from build123d import *

# Parameters (mm, degrees)
SKETCH024_W             = 144.5
SKETCH024_H             = 350
PAD017_DEPTH            = 19
FILLET007_R             = 20
SKETCH025_R             = 2
POCKET015_DEPTH         = 19.001
CHAMFER005_SIZE         = 5
POCKET020_DEPTH         = 19.001
CHAMFER006_SIZE         = 5
CHAMFER007_SIZE         = 3
SKETCH045_W             = 131
SKETCH045_H             = 20
POCKET029_DEPTH         = 14
BODY013_PLACEMENT_ANGLE = 180


with BuildPart() as part:
    # Sketch024 → Pad017 (new body)
    with BuildSketch(Plane.XY):
        with Locations((307.25, 41.2)):
            Rectangle(SKETCH024_W, SKETCH024_H)
    extrude(amount=PAD017_DEPTH)

    # Fillet007
    fillet007_edges = [part.edges().sort_by_distance(p)[0] for p in [
        (379.5, 216.2, 9.5),
        (379.5, -133.8, 9.5),
    ]]
    fillet(fillet007_edges, radius=FILLET007_R)

    # Sketch025 (on Face5 of Fillet007) → Pocket015 (cut, through all)
    with BuildSketch(Plane.XY.offset(19)):
        with Locations((359.5, 196.2)):
            Circle(SKETCH025_R)
        with Locations((359.5, -113.8)):
            Circle(SKETCH025_R)
        with Locations((255, -113.8)):
            Circle(SKETCH025_R)
        with Locations((255, 196.2)):
            Circle(SKETCH025_R)
    extrude(amount=-POCKET015_DEPTH, mode=Mode.SUBTRACT)

    # Chamfer005
    chamfer005_edges = [part.edges().sort_by_distance(p)[0] for p in [
        (297.25, 216.2, 19),
        (235, 41.2, 19),
    ]]
    chamfer(chamfer005_edges, length=CHAMFER005_SIZE)

    # Sketch030 (on Face9 of Chamfer005) → Pocket020 (cut, through all)
    with BuildSketch(Plane.XY.offset(19)):
        with BuildLine():
            Line((256.961524, 95.358984), (276.961524, 130))
            ThreePointArc((311.60254, 110), (295, 121.243557), (276.961524, 130))
            Line((311.60254, 110), (291.60254, 75.358984))
            ThreePointArc((291.60254, 75.358984), (275.286367, 87.098543), (256.961524, 95.358984))
        make_face()
    extrude(amount=-POCKET020_DEPTH, mode=Mode.SUBTRACT)

    # Chamfer006
    chamfer006_edges = [part.edges().sort_by_distance(p)[0] for p in [
        (295, 121.243557, 19),
        (266.961524, 112.679492, 19),
        (275.286367, 87.098543, 19),
        (301.60254, 92.679492, 19),
    ]]
    chamfer(chamfer006_edges, length=CHAMFER006_SIZE)

    # Chamfer007
    chamfer007_edges = [part.edges().sort_by_distance(p)[0] for p in [
        (253, 196.2, 19),
        (357.5, 196.2, 19),
        (357.5, -113.8, 19),
        (253, -113.8, 19),
    ]]
    chamfer(chamfer007_edges, length=CHAMFER007_SIZE)

    # Sketch045 (on Face30 of Chamfer007) → Pocket029 (cut)
    with BuildSketch(Plane(origin=(0, 0, 0), x_dir=(1, 0, 0), z_dir=(0, 0, -1))):
        with Locations((300.5, 98.8)):
            Rectangle(SKETCH045_W, SKETCH045_H)
    extrude(amount=-POCKET029_DEPTH, mode=Mode.SUBTRACT)


with BuildPart() as part_1:
    # Body013 placement: moved
    add(part.part.moved(Location((0, 0, 10))).rotate(Axis((0, 0, 10), (0, 1, 0)), BODY013_PLACEMENT_ANGLE))


solid = part_1.part
Check sheet for the modelled part. Datum: model origin and axes. Units: mm. A direction names the side the tool comes from. Round coordinates to 2 decimals unless told otherwise and drop trailing zeros. Order: outer loops, then holes, each group sorted by start corner. A loop starts at its lowest first (then second) coordinate and runs counter-clockwise, first axis right, second up.
(1) Access from +Z, -Z, +X, -X, +Y, -Y to the whole of each face (thin tool, end or side, straight path). Record for faces 1 (the flat face through (-301.74, 92.92, 2.9)), 2 (the cylindrical face through (-373.797, 210.186, 2.902)), 3 (the flat face through (-366, -99, 3)), 4 (the flat face through (-264.136, 112.716, -6.465)).
(2) Cross-section at A-A, the plane z = -0.75. Enter the section's corners in (x, y).
(3) Cross-section at B-B, the plane x = -333. Enter the section's corners in (y, z), and give its area (4 significant figures).
(4) Draft check along X on faces 5 (the conical face through (-371.24, -125.285, -7.576)), 6 (the flat face through (-300, -99, -4)), 7 (the flat face through (-303.401, 90.864, -6.465)). Enter one of: pulls with the +X half, pulls with the -X half, needs draft (parallel to the pull), parting line crosses it, or undercut.
(5) Go/stop test with flat-tipped pins: P1, Ø16, axis at x = -281, y = -98, coming from the +Z side; P2, Ø6.5, axis at x = -255, y = -113.8, coming from the -Z side. Record where each tip stops, or that it passes through.
(6) Scan lines: probe 1 along Y at (x, z) = (-255, 2.25); probe 2 along X at (y, z) = (196.2, 6.75); probe 3 along Y at (x, z) = (-345, -2). Record each from-to range of solid material in increasing order.
Check sheet entries:
1. face 1: +Z, -Z
1. face 2: +Z, -Z, -X, +Y
1. face 3: +Z, +X
1. face 4: -Z
2. outline: (-379.5, -113.8) arc R20 ccw to (-359.5, -133.8) - (-235, -133.8) - (-235, -108.8) - (-366, -108.8) - (-366, -88.8) - (-235, -88.8) - (-235, 216.2) - (-359.5, 216.2) arc R20 ccw to (-379.5, 196.2) - close; hole circle Ø4 at (-359.5, -113.8); hole circle Ø4 at (-359.5, 196.2); hole (-311.6, 110) - (-291.6, 75.36) arc R100.57 cw to (-256.96, 95.36) - (-276.96, 130) arc R140 ccw to start; hole circle Ø4 at (-255, -113.8); hole circle Ø4 at (-255, 196.2)
3. outline: (-133.8, -4) - (-128.8, -9) - (211.2, -9) - (216.2, -4) - (216.2, 10) - (-88.8, 10) - (-88.8, -4) - (-108.8, -4) - (-108.8, 10) - (-133.8, 10) - close
3. area: 6,345 mm2
4. face 5: pulls with the -X half
4. face 6: needs draft
4. face 7: undercut
5. P1: stops at z = -4
5. P2: stops at z = -7.25
6. probe 1: y = -133.8 to -115.8, -111.8 to -108.8, -88.8 to 194.2, 198.2 to 216.2
6. probe 2: x = -379.5 to -361.5, -357.5 to -257, -253 to -235
6. probe 3: y = -133.8 to -108.8, -88.8 to 216.2
